The listing builds one solid part. Answer for the finished solid, in the listing's coordinates (mm). Face numbers are marked on the shaded views. A direction names the side the tool comes from. Round coordinates to 2 decimals unless told otherwise and drop trailing zeros. Write each loop counter-clockwise with the first axis right and the second up, starting at its lowest first coordinate (ties: lowest second). Pieces come first, ordered by that corner, then holes. Notation, with made-up numbers: M -27.5,20 L 21.5,20 A38 ccw 21.5,58 Z; hole C 74.25,21 d8. An arc over 180 degrees is marked long. One line per item, written item: value. Start each with the question number.
(1) For the marked faces 1 and 2, determine the directions among +Z, -Z, +X, -X, +Y, -Y from which every point of the face is accessible in a straight line to the end or side of a thin tool.
(2) Consider probe 1 along Z at (x, y) = (16, -3.25); probe 2 along X at (y, z) = (-19.5, 13); probe 3 along Z at (x, y) = (9, -11.25). Determine where each line is inside the solid, lowest interval first.
(3) Section A-A (z = 22.75) is taken. Determine the outline of the cut face in (x, y).
(4) Section C-C (x = 12.75) is taken. Determine the outline of the cut face in (y, z), plus the area to 3 significant figures.
(5) Section D-D (y = -17.25) is taken. Determine the outline of the cut face in (x, z), plus the area to 3 significant figures.
(6) Section B-B (y = -11.5) is taken. Determine the outline of the cut face in (x, z), plus the area to 3 significant figures.
(7) Given P1, Ø6, axis at y = -16.5, z = 12.5, coming from the +X side; P2, Ø1.9, axis at y = -12.05, z = 21.98, coming from the -X side, each flat-ended and moving along its own axis, determine where each tip first touches the part or whether it passes through.
```python
from build123d import *

# Parameters (mm, degrees)
F0_W     = 25.4
F0_H     = 25.4
F1_DEPTH = 25.4
F2_W     = 5.039918
F2_H     = 25.4
F3_DEPTH = 38.1
F4_R     = 1.5875
F5_DEPTH = 12.7


with BuildPart() as f1:
    # F0 (on Front) → F1 (new body)
    with BuildSketch(Plane.XZ):
        with Locations((12.7, 12.7)):
            Rectangle(F0_W, F0_H)
    extrude(amount=F1_DEPTH)

    # F2 (on face) → F3 (cut)
    with BuildSketch(Plane.XZ.offset(25.4)):
        Polygon((25.4, 25.4), (9.180619, 25.4), (9.180619, 4.931298), (20.66166, 4.931298), (20.66166, 0), (25.4, 0), align=None)
        with Locations((2.519959, 12.7)):
            Rectangle(F2_W, F2_H)
    extrude(amount=-F3_DEPTH, mode=Mode.SUBTRACT)

    # F4 (on face) → F5 (cut)
    with BuildSketch(Plane(origin=(5.039918, 0, 0), x_dir=(0, -1, 0), z_dir=(-1, 0, 0))):
        with Locations((12.050226, 21.982256)):
            Circle(F4_R)
    extrude(amount=-F5_DEPTH, mode=Mode.SUBTRACT)


solid = f1.part
```
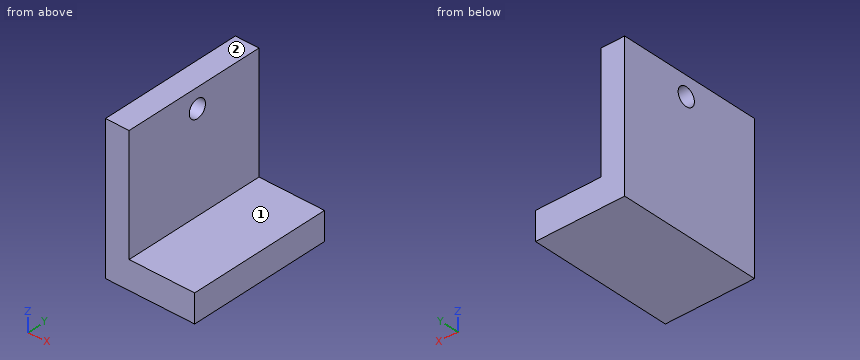
Recorded:
1. face 1: +Z, +X, +Y, -Y
1. face 2: +Z, +X, -X, +Y, -Y
2. probe 1: z = 0 to 4.93
2. probe 2: x = 5.04 to 9.18
2. probe 3: z = 0 to 20.61, 23.35 to 25.4
3. outline: M 5.04,-25.4 L 9.18,-25.4 L 9.18,-13.44 L 5.04,-13.44 Z; M 5.04,-10.66 L 9.18,-10.66 L 9.18,0 L 5.04,0 Z
4. outline: M -25.4,0 L 0,0 L 0,4.93 L -25.4,4.93 Z
4. area: 125 mm2
5. outline: M 5.04,0 L 20.66,0 L 20.66,4.93 L 9.18,4.93 L 9.18,25.4 L 5.04,25.4 Z
5. area: 162 mm2
6. outline: M 5.04,0 L 20.66,0 L 20.66,4.93 L 9.18,4.93 L 9.18,20.49 L 5.04,20.49 Z; M 5.04,23.47 L 9.18,23.47 L 9.18,25.4 L 5.04,25.4 Z
6. area: 149 mm2
7. P1: stops at x = 9.18
7. P2: passes through
